Autodesk Inventor part; units mm, degrees
ref_plane "YZ Plane" through (0, 0, 0) normal (1, 0, 0) x (0, 1, 0)
ref_plane "XZ Plane" through (0, 0, 0) normal (0, 1, 0) x (-1, 0, 0)
ref_plane "XY Plane" through (0, 0, 0) normal (0, 0, 1) x (1, 0, 0)
sketch "Skizze1" plane through (0, 0, 0) normal (0, 0, 1) x (1, 0, 0)
  arc A0 (0, 180) -> (-180, 0) centre (0, 0) ccw
  line L0 (-260.7351, 0) -> (43.4558, 0)
  line L1 (0, -43.4558) -> (0, 260.7351)
  dimension "d0" = 180
  dimension "d1" = 90
sketch "Skizze2" plane through (0, 0, 0) normal (0, 1, 0) x (-1, 0, 0)
  line L0 (0, -42) -> (0, 42)
  circle A0 centre (180, 0) radius 7
  line L1 (252, 0) -> (-42, 0)
  circle A1 centre (180, 0) radius 9
  line L2 (191.9553, 0) -> (171, 0)
  line L3 (173, 0) -> (160, 0)
  line L4 (173, 2) -> (173, 0)
  line L5 (187, 0) -> (200, 0)
  line L6 (187, 2) -> (187, 0)
  circle A2 centre (180, 0) radius 30
  line L7 (187, 2) -> (209.9333, 2)
  line L8 (173, 2) -> (150.0667, 2)
  point P0 (0, 0)
  point P1 (173, 0)
  point P2 (171, 0)
  point P3 (189, 0)
  point P4 (188.775, 2)
  point P5 (171.225, 2)
  point P6 (150, 0)
  point P7 (210, 0)
  dimension "d5" = 18
  dimension "d3" = 180
  dimension "d4" = 14
  dimension "d16" = 60
  dimension "d17" = 2
  dimension "d18" = 23
  dimension "d19" = 7
sweep "Sweeping1" add profiles "Skizze2" path "Skizze1" path curves A0 contours L6 L7 A1 L1 | A0 L4 L8 A1 L7 L6 | L1 A1 L8 L4 | A1 L7 A2 L1 | L1 A2 L8 A1
sketch "Skizze7" plane through (-171.225, 0, 2) normal (0, 0, 1) x (1, 0, 0)
  line L0 (18.1678, 0) -> (18.1678, -3)
  line L1 (0, 0) -> (21.1583, 0)
  line L2 (171.225, 150) -> (171.1678, 150)
  line L3 (171.225, 171.225) -> (171.225, 150.0667)
  line L4 (171.225, 210) -> (171.1678, 210)
  arc A0 (171.225, 150.0667) -> (21.1583, 0) centre (171.225, 0) ccw
  circle A1 centre (171.225, 0) radius 171
  line L5 (-41.8322, 0) -> (-41.8322, -3)
  point P0 (10.1678, 15)
  point P1 (56.0828, 112.085)
  point P2 (156.225, 158)
  point P3 (21.225, 0)
  point P4 (-38.775, 0)
  dimension "d36" = 8
  dimension "d37" = 15
  dimension "d38" = 8
  dimension "d39" = 15
  dimension "d41" = 97.915
  dimension "d42" = 97.915
hole "Bohrung1" at (-161.0572, 15, 2) at (-115.1422, 112.085, 2) at (-15, 158, 2) direction (0, 0, -1) diameter 4 depth 8
sketch "Skizze8" plane through (-209.9333, 0, 2) normal (0, 0, 1) x (1, 0, 0)
  line L0 (-0.0667, 0) -> (-0.0667, -3)
  line L1 (0, 0) -> (21.1583, 0)
  line L2 (209.9333, 209.9333) -> (209.9333, 188.775)
  line L3 (209.9333, 210) -> (212.9333, 210)
  arc A0 (209.9333, 171.225) -> (38.7082, 0) centre (209.9333, 0) ccw
  circle A1 centre (209.9333, 0) radius 200.8827
  point P0 (9.6113, 15)
  point P1 (67.8861, 142.044)
  point P2 (194.9333, 200.3219)
  dimension "d51" = 15
  dimension "d52" = 15
  dimension "d54" = 142.044
  dimension "d59" = 401.7655
  dimension "d60" = 142.0471
hole "Bohrung3" at (-200.3219, 15, 2) at (-142.0471, 142.044, 2) at (-15, 200.3219, 2) direction (0, 0, -1) diameter 4 depth 8
properties part number "Kurventeil-Ph-L-dünn"
Verification items for the finished model (mm, model axes). A direction names the side the tool comes from. Give positions to 0.01 mm unless a question says otherwise; leave off trailing zeros. Loops run counter-clockwise (first coordinate to the right, second up) from the corner with the lowest first, then second, coordinate; pieces in that order, holes last.
1. Set-up check for faces 1 (the flat face through (-135, 136, 2)), 2 (the flat face through (-112, 101, 2)), 3 (the flat face through (-179.86, 0, 7.15)): record each of +Z, -Z, +X, -X, +Y, -Y from which the full face is reachable in a straight line by a thin tool's end or side.
2. Section check A-A, the plane z = 4.75. Enter the section's corners in (x, y).
3. Thickness scan on line 1 (Y direction, x = -15, z = 0.7); line 2 (Y direction, x = -15, z = 1.6); line 3 (Z direction, x = -150, y = 11). Record the ranges inside material, lowest first.
4. Go/stop test with flat-tipped pins: pin 1 Ø4.5 at (x, y) = (-142.05, 142.04) entering from -Z; pin 2 Ø5 at (x, z) = (-132.5, 1.5) entering from -Y; pin 3 Ø4 at (y, z) = (44, 3) entering from -X; pin 4 Ø3 at (x, y) = (-149.5, 110) entering from +Z. Record where each tip stops, or that it passes through.
Geometry says:
1. face 1: +Z, -X, +Y
1. face 2: +Z, +X, -Y
1. face 3: +Z, -Z, +X, -X, -Y
2. outline: (-187.64, 0) - (-185.14, 0) arc R185.14 cw to (0, 185.14) - (0, 187.64) arc R187.64 ccw to start; (-174.86, 0) - (-172.36, 0) arc R172.36 cw to (0, 172.36) - (0, 174.86) arc R174.86 ccw to start
3. line 1: y = 149.26 to 156, 160 to 172.38, 186.36 to 198.32, 202.32 to 209.46
3. line 2: y = 149.29 to 156, 160 to 172.53, 186.21 to 198.32, 202.32 to 209.42
3. line 3: z = 0 to 2
4. pin 1: stops at z = 0
4. pin 2: stops at y = 65.46
4. pin 3: stops at x = -205.63
4. pin 4: stops at z = 8.01
